```python
from build123d import *

# Parameters (mm, degrees)
EXTRUDE_1_DEPTH = 20
SKETCH_3_W      = 54
SKETCH_3_H      = 62
EXTRUDE_2_DEPTH = 58


with BuildPart() as part:
    # Эскиз2 → Бобышка-Вытянуть1 (new body)
    with BuildSketch(Plane(origin=(0, 0, 0), x_dir=(1, 0, 0), z_dir=(0, 1, 0))):
        with BuildLine():
            Line((-37, -31), (37, -31))
            ThreePointArc((37, -31), (45.485281374, -27.485281374), (49, -19))
            Line((49, -19), (49, 19))
            ThreePointArc((49, 19), (45.485281374, 27.485281374), (37, 31))
            Line((37, 31), (-37, 31))
            ThreePointArc((-37, 31), (-45.485281374, 27.485281374), (-49, 19))
            Line((-49, 19), (-49, -19))
            ThreePointArc((-49, -19), (-45.485281374, -27.485281374), (-37, -31))
        make_face()
    extrude(amount=EXTRUDE_1_DEPTH)

    # Эскиз3 → Бобышка-Вытянуть2 (add)
    with BuildSketch(Plane(origin=(0, 20, 0), x_dir=(1, 0, 0), z_dir=(0, 1, 0))):
        Rectangle(SKETCH_3_W, SKETCH_3_H)
    extrude(amount=EXTRUDE_2_DEPTH)


solid = part.part
```
Check sheet for the modelled part. Datum: model origin and axes. Units: mm. A direction names the side the tool comes from. Round coordinates to 2 decimals unless told otherwise and drop trailing zeros. Order: outer loops, then holes, each group sorted by start corner. A loop starts at its lowest first (then second) coordinate and runs counter-clockwise, first axis right, second up. Notation, with made-up numbers: (-19.5, 64.25) -> (27.5, 64.25) arc R11 cw to (27.5, 71.25) -> close; hole circle Ø1 at (-38.75, -39.75). An arc over 180 degrees is marked (long way). One line per item, written item: value. Start each with the question number.
Q1. Cross-section at A-A (z = 1.5). Record the boundary of the cut face in (x, y), and give its area (3 significant figures).
Q2. Thickness scan on line 1 (X direction, y = 49.5, z = -21); line 2 (Y direction, x = 33.5, z = -16); line 3 (Z direction, x = 39, y = 16). Record the ranges inside material, lowest first.
Q3. Cross-section at B-B (y = 14). Record the boundary of the cut face in (x, z).
Q4. Cross-section at D-D (y = 24). Record the boundary of the cut face in (x, z), and give its area (3 significant figures).
Q5. Cross-section at C-C (x = -32). Record the boundary of the cut face in (y, z), and give its area (3 significant figures).
Q6. Gauge pin test, flat ends, axial feed: pin 1 Ø2 at (y, z) = (24.5, 7.5) entering from +X; pin 2 Ø11 at (x, z) = (-43, 3) entering from +Y. Record the tip position at first contact, or that the pin passes through.
Q7. Set-up check for faces 1 (the face through (-27, 49, 0)), 2 (the face through (38, 20, 0)), 3 (the face through (-45.39, 9.86, -27.58)): record each of +Z, -Z, +X, -X, +Y, -Y from which the full face is reachable in a straight line by a thin tool's end or side.
Completed:
1. outline: (-49, 0) -> (49, 0) -> (49, 20) -> (27, 20) -> (27, 78) -> (-27, 78) -> (-27, 20) -> (-49, 20) -> close
1. area: 5,090 mm²
2. line 1: x = -27 to 27
2. line 2: y = 0 to 20
2. line 3: z = -30.83 to 30.83
3. outline: (-49, -19) arc R12 ccw to (-37, -31) -> (37, -31) arc R12 ccw to (49, -19) -> (49, 19) arc R12 ccw to (37, 31) -> (-37, 31) arc R12 ccw to (-49, 19) -> close
4. outline: (-27, -31) -> (27, -31) -> (27, 31) -> (-27, 31) -> close
4. area: 3,350 mm²
5. outline: (0, -31) -> (20, -31) -> (20, 31) -> (0, 31) -> close
5. area: 1,240 mm²
6. pin 1: stops at x = 27
6. pin 2: stops at y = 20
7. face 1: +Z, -Z, -X, +Y
7. face 2: +Z, -Z, +X, +Y
7. face 3: -Z, -X, +Y, -Y
